Design review of the part built by this model. Coordinates are the model's own, in mm. A direction names the side the tool comes from. Round coordinates to 2 decimals unless told otherwise and drop trailing zeros. Order: outer loops, then holes, each group sorted by start corner. A loop starts at its lowest first (then second) coordinate and runs counter-clockwise, first axis right, second up. Notation, with made-up numbers: (78, 53.5) - (96, 53.5) arc R30 cw to (96, 75.5) - close; hole circle Ø5 at (-8.75, 34.25). An arc over 180 degrees is marked (long way). Answer as a JSON object with one key per item and string values. Group by question number.
from build123d import *

# Parameters (mm, degrees)
BOSS_EXTRUDE1_DEPTH = 3
BOSS_EXTRUDE2_DEPTH = 24.4
BOSS_EXTRUDE3_DEPTH = 3
CUT_EXTRUDE2_DEPTH  = 101
CUT_EXTRUDE3_DEPTH  = 101


with BuildPart() as part:
    # Sketch1 → Boss-Extrude1 (new body)
    with BuildSketch(Plane(origin=(0, 0, 0), x_dir=(1, 0, 0), z_dir=(0, 1, 0))):
        Polygon((0, 0), (0, 100), (20, 100), (20, 20), (100, 20), (100, 0), align=None)
    extrude(amount=BOSS_EXTRUDE1_DEPTH)

    # Sketch2 → Boss-Extrude2 (add)
    with BuildSketch(Plane(origin=(0, 3, 0), x_dir=(1, 0, 0), z_dir=(0, 1, 0))):
        Polygon((0, 100), (0, 0), (100, 0), (100, 5), (5, 5), (5, 100), align=None)
    extrude(amount=BOSS_EXTRUDE2_DEPTH)

    # Sketch3 → Boss-Extrude3 (add)
    with BuildSketch(Plane(origin=(0, 27.4, 0), x_dir=(1, 0, 0), z_dir=(0, 1, 0))):
        Polygon((0, 0), (0, 60), (5, 60), (60, 5), (60, 0), align=None)
    extrude(amount=BOSS_EXTRUDE3_DEPTH)

    # Sketch4 → Cut-Extrude2 (cut, through all)
    with BuildSketch(Plane.ZY):
        Polygon((-60, 27.4), (-100, 3), (-100, 27.4), align=None)
    extrude(amount=-CUT_EXTRUDE2_DEPTH, mode=Mode.SUBTRACT)

    # Sketch5 → Cut-Extrude3 (cut, through all)
    with BuildSketch(Plane.XY):
        Polygon((60, 27.4), (100, 3), (100, 27.4), align=None)
    extrude(amount=-CUT_EXTRUDE3_DEPTH, mode=Mode.SUBTRACT)


solid = part.part
1. Clearance check with flat-ended pins moving along their axes: P1, Ø12, axis at x = 47.5, y = 24, coming from the +Z side; P2, Ø1.5, axis at x = 40.5, y = 2, coming from the -Z side; P3, Ø0.9, axis at y = 2, z = -80, coming from the +X side; P4, Ø5, axis at y = 13, z = -36, coming from the +X side. State where each tip first meets the part, or that it passes through.
2. Take a section at C-C, the plane x = 67. Give the boundary of the cut face in (y, z).
3. To check wall thickness, follow line 1 (Y direction, x = 10, z = -19.5); line 2 (Y direction, x = 34, z = -23); line 3 (X direction, y = 12, z = -65). State the ranges of each line that lie inside material, in increasing order. Write a range as from..to.
4. Take a section at B-B, the plane z = -44.5. Give the boundary of the cut face in (x, y), then the cut area to 4 significant figures.
5. Tool access review of faces 1 (the flat face through (18, 3, -35)), 2 (the flat face through (2, 29, -60)), 3 (the flat face through (20, 1, -61)): name each direction out of +Z, -Z, +X, -X, +Y, -Y from which nothing blocks a thin tool from reaching the whole face with its end or side.
6. Mouldability with a two-part tool opening along Y and no side actions: class faces 4 (the flat face through (79.72, 15.37, -2.46)), 5 (the flat face through (43, 15, -5)), 6 (the flat face through (40, 15, 0)) as pulls with the +Y half, pulls with the -Y half, needs draft (parallel to the pull), parting line crosses it, or undercut.
7. Take a section at D-D, the plane y = 5. Give the boundary of the cut face in (x, z).
8. Take a section at A-A, the plane x = 50.5. Give the boundary of the cut face in (y, z).
Response values:
{
 "1": {"P1": "z = 0", "P2": "z = -20", "P3": "x = 20", "P4": "x = 5"},
 "2": {"outline": "(0, -20) - (3, -20) - (3, -5) - (23.13, -5) - (23.13, 0) - (0, 0) - close"},
 "3": {"line 1": "0..3, 27.4..30.4", "line 2": "27.4..30.4", "line 3": "0..5"},
 "4": {"outline": "(0, 0) - (20, 0) - (20, 3) - (5, 3) - (5, 27.4) - (20.5, 27.4) - (20.5, 30.4) - (0, 30.4) - close", "area": "243.5 mm2"},
 "5": {"face 1": "-Z, +X", "face 2": "-Z, +X, -X, +Y", "face 3": "-Z, +X, -Y"},
 "6": {"face 4": "pulls with the +Y half", "face 5": "undercut", "face 6": "needs draft"},
 "7": {"outline": "(0, -96.72) - (5, -96.72) - (5, -5) - (96.72, -5) - (96.72, 0) - (0, 0) - close"},
 "8": {"outline": "(0, -20) - (3, -20) - (3, -5) - (27.4, -5) - (27.4, -14.5) - (30.4, -14.5) - (30.4, 0) - (0, 0) - close"}
}
